```python
from build123d import *

# Parameters (mm, degrees)
F0_W          = 25
F0_H          = 25
F1_DEPTH      = 25
F3_DEPTH      = 12.501
F3_DEPTH_BACK = 12.501
F5_DEPTH      = 12.501
F5_DEPTH_BACK = 12.501


with BuildPart() as f1:
    # F0 (on Top) → F1 (new body)
    with BuildSketch(Plane.XY):
        Rectangle(F0_W, F0_H)
    extrude(amount=F1_DEPTH)

    # F2 (on Right) → F3 (cut, two sides)
    with BuildSketch(Plane.YZ) as f3_sk:
        Polygon((0, 12.5), (12.5, 0), (12.5, 25), (-12.5, 25), (-12.5, 0), align=None)
    extrude(amount=-F3_DEPTH, mode=Mode.SUBTRACT)
    extrude(f3_sk.sketch, amount=F3_DEPTH_BACK, mode=Mode.SUBTRACT)

    # F4 (on Front) → F5 (cut, two sides)
    with BuildSketch(Plane.XZ) as f5_sk:
        Polygon((0, 12.5), (12.5, 0), (12.5, 25), (-12.5, 25), (-12.5, 0), align=None)
    extrude(amount=-F5_DEPTH, mode=Mode.SUBTRACT)
    extrude(f5_sk.sketch, amount=F5_DEPTH_BACK, mode=Mode.SUBTRACT)


solid = f1.part
```
Build history of the part. All positions in model axes, mm. Give positions to 0.01 mm unless a question says otherwise; leave off trailing zeros. Loops run counter-clockwise (first coordinate to the right, second up) from the corner with the lowest first, then second, coordinate; pieces in that order, holes last. Notation, with made-up numbers: (86.5, -34.5) -> (116.5, -34.5) arc R25 cw to (116.5, -19.5) -> close; hole circle Ø8 at (41.5, 71.5). An arc over 180 degrees is marked (long way). One line per question, with ' | ' between items. Start each with the question number.
1) Pin check, flat tips, straight feed: pin 1 (2 mm diameter, centred on x = -5, y = 2.5, fed in from +Z); pin 2 (2 mm diameter, centred on x = -1, z = 5.5, fed in from -Y); pin 3 (1.5 mm diameter, centred on y = -9, z = 1.5, fed in from -X); pin 4 (1.5 mm diameter, centred on x = -4.5, z = 11, fed in from -Y). Stop position of each tip, or through.
2) Cut at A-A (x = 7.5). Give the cut face in (y, z), plus the area to 3 significant figures.
3) Probe L1, parallel to Z at x = 0, y = -3.75; L2, parallel to Y at x = -1.5, z = 10.75; L3, parallel to Z at x = -8.75, y = -6.25. List the from-to ranges inside material, lowest first.
4) Cut at B-B (z = 6.75). Give the cut face in (x, y), plus the area to 3 significant figures.
Return value:
1) pin 1: z = 8.5 | pin 2: y = -8 | pin 3: x = -11.75 | pin 4: through
2) outline: (-12.5, 0) -> (12.5, 0) -> (7.5, 5) -> (-7.5, 5) -> close | area: 100 mm^2
3) L1: 0 to 8.75 | L2: -1.75 to 1.75 | L3: 0 to 3.75
4) outline: (-5.75, -5.75) -> (5.75, -5.75) -> (5.75, 5.75) -> (-5.75, 5.75) -> close | area: 132 mm^2
